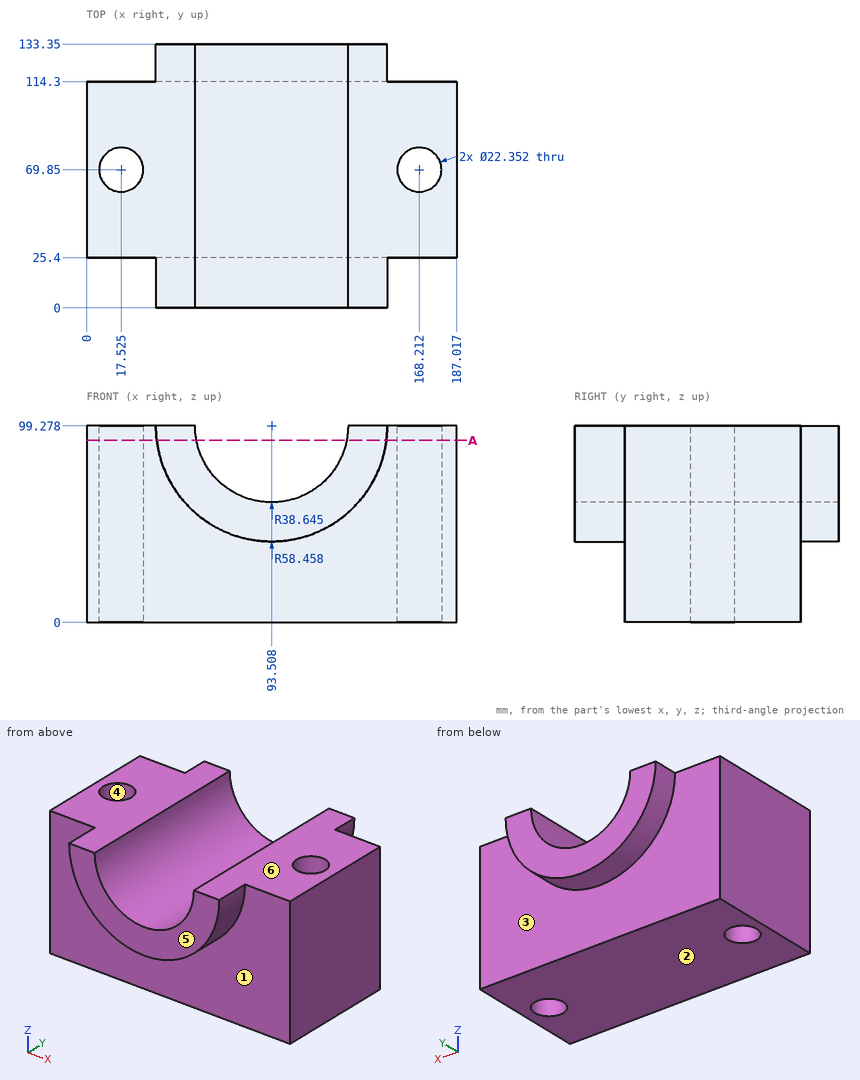
Study the drawing (mm; zero at the part's minimum x, y, z) and answer. A direction names the side the tool comes from. Coordinates: 2 decimals unless noted, no trailing zeros. Answer in a Markdown table with one row per item. Add a question column.
Item 1: Which of the six approach directions +Z, -Z, +X, -X, +Y, -Y give full straight-line access (tool end or side, diameter ignored) to the marked faces 1, 2 and 3?
Item 2: Find the intervals of material crossed by L1, parallel to X at y = 69, z = 37 (1 decimal); L2, parallel to Y at x = 63.5, z = 16.5; L3, parallel to Z at x = 92.5, y = 12 (1 decimal), in increasing order. Write a range as from..to.
Item 3: Each of these flat-tipped pins is pushed along its axis until it touches: P1, Ø12, axis at x = 147.5, z = 19.5, coming from the +Y side; P2, Ø1.5, axis at x = 69.5, y = 105, coming from the +Z side (1 decimal). Where does it stop, or does it pass through?
Item 4: Find section A-A (z = 92). State how many separate pieces and enclosed holes the cut face has, then the cut area to 3 significant figures.
Item 5: Determine the mould class of the marked faces 4, 5 and 6 for opening direction Y: +Y half, -Y half, draft (parallel to the pull), parting line (faces both ways), or undercut.
Result set:
| question | item | result |
|---|---|---|
| 1 | face 1 | -Z, -Y |
| 1 | face 2 | -Z, +X, -X, +Y, -Y |
| 1 | face 3 | -Z, +Y |
| 2 | L1 | x = 0..6.4, 28.7..157.1, 179.4..187 |
| 2 | L2 | y = 25.4..114.3 |
| 2 | L3 | z = 40.8..60.6 |
| 3 | P1 | stops at y = 114.3 |
| 3 | P2 | stops at z = 69.6 |
| 4 | separate pieces | 2 |
| 4 | enclosed holes | 2 |
| 4 | area | 10,900 mm² |
| 5 | face 4 | undercut |
| 5 | face 5 | -Y half |
| 5 | face 6 | draft |
